from build123d import *

# Parameters (mm, degrees)
SKETCH1_R           = 1.7
BOSS_EXTRUDE1_DEPTH = 3.8


with BuildPart() as part:
    # Sketch1 → Boss-Extrude1 (new body)
    with BuildSketch(Plane.XY):
        with BuildLine():
            Line((-170.500000005, 25.75), (-88.925688775, 25.75))
            ThreePointArc((-88.925688775, 25.75), (-77.757832362, 14.582143587), (-66.589975949, 25.75))
            Line((-66.589975949, 25.75), (66.589975949, 25.75))
            ThreePointArc((66.589975949, 25.75), (77.757832362, 14.582143587), (88.925688775, 25.75))
            Line((88.925688775, 25.75), (170.500000005, 25.75))
            Line((170.500000005, 25.75), (170.500000005, 45.331584009))
            Line((170.500000005, 45.331584009), (50.500000005, 64.913168018))
            ThreePointArc((50.500000005, 64.913168018), (0, 115.413168023), (-50.500000005, 64.913168018))
            Line((-50.500000005, 64.913168018), (-170.500000005, 45.331584009))
            Line((-170.500000005, 45.331584009), (-170.500000005, 25.75))
        make_face()
        with Locations(Location((15.95, 71.613168018, 0), (0, 0, 180))):
            Circle(SKETCH1_R, mode=Mode.SUBTRACT)
        with Locations(Location((7.975, 57.800062828, 0), (0, 0, 180))):
            Circle(SKETCH1_R, mode=Mode.SUBTRACT)
        with Locations(Location((-7.975, 57.800062828, 0), (0, 0, 180))):
            Circle(SKETCH1_R, mode=Mode.SUBTRACT)
        with Locations(Location((-15.95, 71.613168018, 0), (0, 0, 180))):
            Circle(SKETCH1_R, mode=Mode.SUBTRACT)
        with Locations(Location((7.975, 85.426273209, 0), (0, 0, 180))):
            Circle(SKETCH1_R, mode=Mode.SUBTRACT)
        with Locations(Location((-7.975, 85.426273209, 0), (0, 0, 180))):
            Circle(SKETCH1_R, mode=Mode.SUBTRACT)
    extrude(amount=BOSS_EXTRUDE1_DEPTH)


solid = part.part
The listing builds one solid part. Answer for the finished solid, in the listing's coordinates (mm). Give positions to 0.01 mm unless a question says otherwise; leave off trailing zeros. Order: outer loops, then holes, each group sorted by start corner. A loop starts at its lowest first (then second) coordinate and runs counter-clockwise, first axis right, second up. Notation, with made-up numbers: (35, -33.75) - (87, -33.75) arc R31 ccw to (87, 2.25) - close; hole circle Ø8 at (26.5, -36.75). An arc over 180 degrees is marked (long way). One line per item, written item: value. Start each with the question number.
1) The mould has two halves that part along X. Classify faces 1 (the face through (-109.66, 55.26, 1.87)), 2 (the face through (-78.003, 14.585, 1.873)), 3 (the face through (77.512, 14.585, 1.873)), 4 (the face through (1.1, 115.4, 1.9)): released by +X, released by -X, zero draft, split by the parting line, or undercut.
2) A cutting plane is placed at C-C on x = -63.5. Give the vertices of the cut face in (y, z).
3) A cutting plane is placed at A-A on z = 2.1. Give the vertices of the cut face in (x, y) (3 decimals), then the cut area to 3 significant figures.
4) A cutting plane is placed at B-B on x = 0. Give the vertices of the cut face in (y, z).
5) Find the intervals of material crossed by L1, parallel to X at y = 71.5, z = 2.95; L2, parallel to Y at x = -15.95, z = 1.65; L3, parallel to X at y = 66, z = 1.6, in increasing order.
6) Given pin 1 Ø2 at (y, z) = (77.5, 2) entering from +X; pin 2 Ø1.1 at (x, z) = (-32, 2.5) entering from -Y; pin 3 Ø1 at (y, z) = (81, 1) entering from +X, each flat-ended and moving along its own axis, determine where each tip first touches the part or whether it passes through.
Answer sheet:
1. face 1: released by -X
1. face 2: undercut
1. face 3: undercut
1. face 4: split by the parting line
2. outline: (25.75, 0) - (62.79, 0) - (62.79, 3.8) - (25.75, 3.8) - close
3. outline: (-170.5, 25.75) - (-88.926, 25.75) arc R11.168 ccw to (-66.59, 25.75) - (66.59, 25.75) arc R11.168 ccw to (88.926, 25.75) - (170.5, 25.75) - (170.5, 45.332) - (50.5, 64.913) arc R50.5 ccw to (-50.5, 64.913) - (-170.5, 45.332) - close; hole circle Ø3.4 at (-15.95, 71.613); hole circle Ø3.4 at (-7.975, 57.8); hole circle Ø3.4 at (-7.975, 85.426); hole circle Ø3.4 at (7.975, 57.8); hole circle Ø3.4 at (7.975, 85.426); hole circle Ø3.4 at (15.95, 71.613)
3. area: 15,300 mm2
4. outline: (25.75, 0) - (115.41, 0) - (115.41, 3.8) - (25.75, 3.8) - close
5. L1: x = -50.07 to -17.65, -14.25 to 14.25, 17.65 to 50.07
5. L2: y = 25.75 to 69.91, 73.31 to 112.83
5. L3: x = -50.49 to 50.49
6. pin 1: stops at x = 49.15
6. pin 2: stops at y = 25.75
6. pin 3: stops at x = 48.03
